from build123d import *

# Parameters (mm, degrees)
SKETCH1_W           = 173.99
SKETCH1_H           = 177.8
BOSS_EXTRUDE1_DEPTH = 3.175
SKETCH3_W           = 12.7
SKETCH3_H           = 3.175
SKETCH3_W_2         = 3.175
SKETCH3_H_2         = 12.7
CUT_EXTRUDE1_DEPTH  = 3.175


with BuildPart() as part:
    # Sketch1 → Boss-Extrude1 (new body)
    with BuildSketch(Plane(origin=(0, 0, 0), x_dir=(1, 0, 0), z_dir=(0, 1, 0))):
        Rectangle(SKETCH1_W, SKETCH1_H)
    extrude(amount=BOSS_EXTRUDE1_DEPTH)

    # Sketch3 → Cut-Extrude1 (cut)
    with BuildSketch(Plane(origin=(0, 3.175, 0), x_dir=(1, 0, 0), z_dir=(0, 1, 0))):
        with Locations((-64.77, 87.3125)):
            Rectangle(SKETCH3_W, SKETCH3_H)
        with Locations((-39.37, 87.3125)):
            Rectangle(SKETCH3_W, SKETCH3_H)
        with Locations((-13.97, 87.3125)):
            Rectangle(SKETCH3_W, SKETCH3_H)
        with Locations((11.43, 87.3125)):
            Rectangle(SKETCH3_W, SKETCH3_H)
        with Locations((36.83, 87.3125)):
            Rectangle(SKETCH3_W, SKETCH3_H)
        with Locations((62.23, 87.3125)):
            Rectangle(SKETCH3_W, SKETCH3_H)
        with Locations((-85.4075, 28.575)):
            Rectangle(SKETCH3_W_2, SKETCH3_H_2)
        with Locations((-85.4075, 53.975)):
            Rectangle(SKETCH3_W_2, SKETCH3_H_2)
        with Locations((-85.4075, 3.175)):
            Rectangle(SKETCH3_W_2, SKETCH3_H_2)
        with Locations((-85.4075, -22.225)):
            Rectangle(SKETCH3_W_2, SKETCH3_H_2)
        with Locations((-85.4075, -47.625)):
            Rectangle(SKETCH3_W_2, SKETCH3_H_2)
        with Locations((-85.4075, -73.025)):
            Rectangle(SKETCH3_W_2, SKETCH3_H_2)
        with Locations((85.4075, -73.025)):
            Rectangle(SKETCH3_W_2, SKETCH3_H_2)
        with Locations((85.4075, -47.625)):
            Rectangle(SKETCH3_W_2, SKETCH3_H_2)
        with Locations((85.4075, -22.225)):
            Rectangle(SKETCH3_W_2, SKETCH3_H_2)
        with Locations((85.4075, 3.175)):
            Rectangle(SKETCH3_W_2, SKETCH3_H_2)
        with Locations((85.4075, 28.575)):
            Rectangle(SKETCH3_W_2, SKETCH3_H_2)
        with Locations((85.4075, 53.975)):
            Rectangle(SKETCH3_W_2, SKETCH3_H_2)
    extrude(amount=-CUT_EXTRUDE1_DEPTH, mode=Mode.SUBTRACT)


solid = part.part
The listing builds one solid part. Answer for the finished solid, in the listing's coordinates (mm). Coordinates: 2 decimals unless noted, no trailing zeros. Write each loop counter-clockwise with the first axis right and the second up, starting at its lowest first coordinate (ties: lowest second). Pieces come first, ordered by that corner, then holes. Notation, with made-up numbers: (-6, -1) - (40, -1) arc R10 cw to (40, 10) - close; hole circle Ø4 at (88.5, 36). An arc over 180 degrees is marked (long way). Answer as CSV lines item,"result".
1. Straight lines are drawn through the part: line 1 (Z direction, x = -14, y = 1.9) (3 decimals); line 2 (X direction, y = 1.35, z = -57). For each, find the intervals that lie inside material, in ascending order. Write a range as [from, to].
Computed values:
line 1,"z = [-85.725, 88.9]"
line 2,"x = [-83.82, 83.82]"
2. Find section B-B (x = 64). Give the vertices of the cut face in (y, z) (3 decimals).
Computed values:
outline,"(0, -85.725) - (3.175, -85.725) - (3.175, 88.9) - (0, 88.9) - close"
3. Find section A-A (z = 46). Give the vertices of the cut face in (x, y) (3 decimals).
Computed values:
outline,"(-83.82, 0) - (83.82, 0) - (83.82, 3.175) - (-83.82, 3.175) - close"
4. Given P1, Ø1, axis at y = 1, z = -5, coming from the +X side, flat-ended and moving along its own axis, determine where the tip first touches the part or whether it passes through.
Computed values:
P1,"stops at x = 83.82"
